Job drawing, mm, ordinate dimensions from the low corner. One solid piece. A direction names the side the tool comes from. Coordinates: 2 decimals unless noted, no trailing zeros. Order: outer loops, then holes, each group sorted by start corner. A loop starts at its lowest first (then second) coordinate and runs counter-clockwise, first axis right, second up. Notation, with made-up numbers: (11, 41.25) - (61, 41.25) arc R13 cw to (61, 49.25) - close; hole circle Ø8 at (-13.5, 44). An arc over 180 degrees is marked (long way). Use a Markdown table: item, result. Add a question column.
1) Saw through at B-B on z = 90. List the corners of the cut face in (x, y), then the cut area to 3 significant figures.
2) Saw through at C-C on y = 46. List the corners of the cut face in (x, z), then the cut area to 3 significant figures.
3) Saw through at A-A on x = 90. List the corners of the cut face in (y, z), then the cut area to 3 significant figures.
4) Tool access for the marked faces 1 and 2: list every direction of +Z, -Z, +X, -X, +Y, -Y with a clear straight run to the whole face (end or side of a thin tool).
5) Saw through at D-D on y = 69. List the corners of the cut face in (x, z).
6) Wall check: L1, parallel to Y at x = 22, z = 138.5; L2, parallel to Y at x = 90, z = 123.5; L3, parallel to X at y = 107, z = 127.5. Give the ranges that are in metal, low to high. Write a range as [from, to].
7) Drop flat-ended pins along their axis: P1, Ø12, axis at y = 57, z = 45.5, coming from the -X side; P2, Ø1, axis at y = 35, z = 126, coming from the -X side; P3, Ø1.5, axis at y = 33.5, z = 81, coming from the -X side; P4, Ø4, axis at x = 151.5, z = 140, coming from the -Y side. Give the stop position or say it passes through.
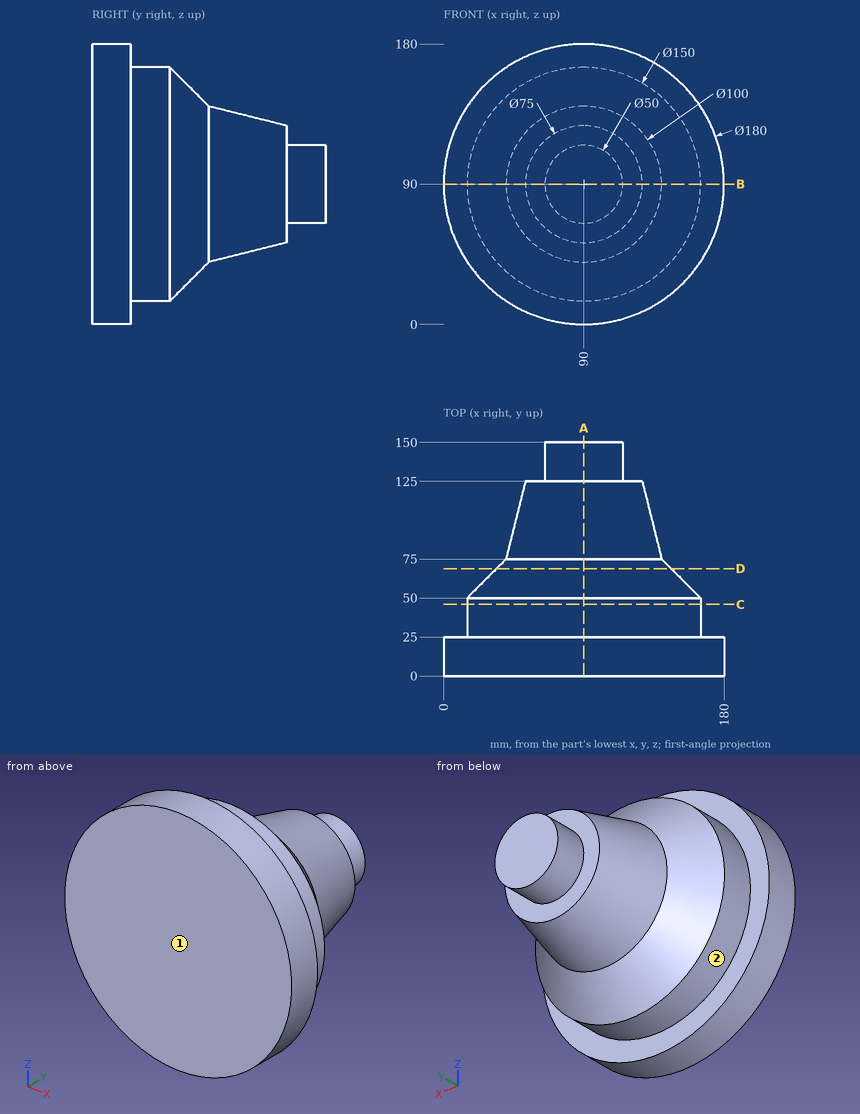
Results are:
| question | item | result |
|---|---|---|
| 1 | outline | (0, 0) - (180, 0) - (180, 25) - (165, 25) - (165, 50) - (140, 75) - (127.5, 125) - (115, 125) - (115, 150) - (65, 150) - (65, 125) - (52.5, 125) - (40, 75) - (15, 50) - (15, 25) - (0, 25) - close |
| 1 | area | 17,000 mm2 |
| 2 | outline | circle Ø150 at (90, 90) |
| 2 | area | 17,700 mm2 |
| 3 | outline | (0, 0) - (25, 0) - (25, 15) - (50, 15) - (75, 40) - (125, 52.5) - (125, 65) - (150, 65) - (150, 115) - (125, 115) - (125, 127.5) - (75, 140) - (50, 165) - (25, 165) - (25, 180) - (0, 180) - close |
| 3 | area | 17,000 mm2 |
| 4 | face 1 | +Z, -Z, +X, -X, -Y |
| 4 | face 2 | +Y |
| 5 | outline | circle Ø112 at (90, 90) |
| 6 | L1 | [0, 25] |
| 6 | L2 | [0, 125] |
| 6 | L3 | [71.09, 108.91] |
| 7 | P1 | x = 29.71 |
| 7 | P2 | x = 23.93 |
| 7 | P3 | x = 15.46 |
| 7 | P4 | y = 0 |
